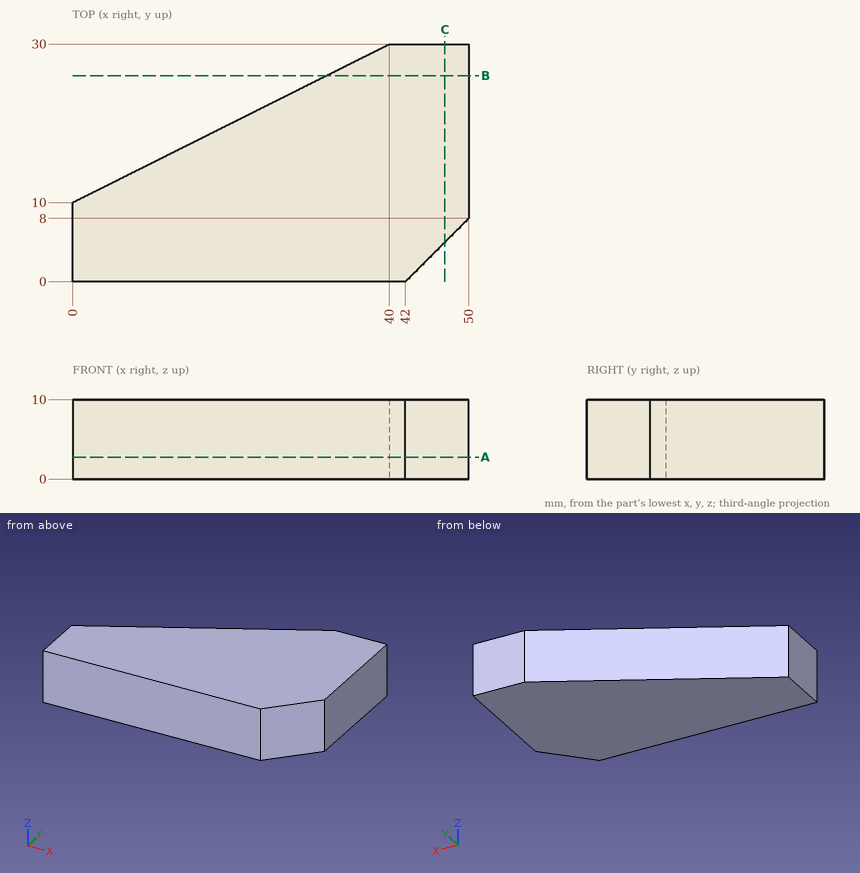
Source: three-view drawing plus pictorial views. Frame: mm from the lowest corner of the part. Coordinates: 2 decimals unless noted, no trailing zeros. Order: outer loops, then holes, each group sorted by start corner. A loop starts at its lowest first (then second) coordinate and runs counter-clockwise, first axis right, second up.
Item 1: Cut plane A-A (z = 2.75). Return loops of the section in (x, y).
Output values:
outline: (0, 0) - (42, 0) - (50, 8) - (50, 30) - (40, 30) - (0, 10) - close
Item 2: First-contact query: P1, Ø6, axis at x = 11.5, z = 5, coming from the +Y side; P2, Ø4, axis at x = 18, z = 1, coming from the -Y side; P3, Ø4, axis at y = 16, z = 4, coming from the -X side. Flat tips, straight axial feed; report the tip coordinate or a pass-through.
Output values:
P1: stops at y = 17.25
P2: stops at y = 0
P3: stops at x = 8
Item 3: Cut plane B-B (y = 26). Return loops of the section in (x, z).
Output values:
outline: (32, 0) - (50, 0) - (50, 10) - (32, 10) - close
Item 4: Material intervals for line 1 (Y direction, x = 35, z = 1.75); line 2 (X direction, y = 6, z = 1.25); line 3 (Y direction, x = 25, z = 5.25), sorted ascending.
Output values:
line 1: y = 0 to 27.5
line 2: x = 0 to 48
line 3: y = 0 to 22.5
Item 5: Cut plane C-C (x = 47). Return loops of the section in (y, z), plus the area to 3 significant figures.
Output values:
outline: (5, 0) - (30, 0) - (30, 10) - (5, 10) - close
area: 250 mm2
